The model under review builds one solid part; all positions refer to its coordinate system, in mm. Face numbers are marked on the shaded views. A direction names the side the tool comes from. Round coordinates to 2 decimals unless told otherwise and drop trailing zeros. Order: outer loops, then holes, each group sorted by start corner. A loop starts at its lowest first (then second) coordinate and runs counter-clockwise, first axis right, second up. Notation, with made-up numbers: M 21,6.5 L 32,6.5 A19 ccw 32,19.5 Z; hole C -21,36.25 d11. An arc over 180 degrees is marked long. Answer as a JSON object with one key per item and string values. Group by question number.
1) Consider section B-B, the plane z = 27.5. Write out the cut boundary in (x, y).
2) Consider section A-A, the plane y = -325.5. Write out the cut boundary in (x, z), then the cut area to 3 significant figures.
3) For the marked faces 1 and 2, list the 3-axis set-ups (+Z, -Z, +X, -X, +Y, -Y) from which the entire face can be reached by the end or side of a thin tool; tool diameter is ignored.
4) Insertion check: pin 1 Ø1 at (y, z) = (247.5, 47) entering from +X; pin 2 Ø4 at (x, y) = (27, 71.5) entering from -Z; pin 3 Ø8 at (x, y) = (7.5, -109.5) entering from -Z. Each pin has a flat end and moves straight along its axis. Give the tip position at first contact, or say it passes through.
5) Consider section C-C, the plane x = 48. Write out the cut boundary in (y, z).
6) To check wall thickness, follow line 1 (X direction, y = -69, z = 53); line 2 (Z direction, x = 9, y = -290); line 3 (X direction, y = -324.5, z = 4). State the ranges of each line that lie inside material, in increasing order.
```python
from build123d import *

# Parameters (mm, degrees)
F1_DEPTH = 482.6
F3_DEPTH = 6.351
F5_R     = 5.08
F4_R     = 7.14375
F6_DEPTH = 101.6


with BuildPart() as f1:
    # F0 (on Front) → F1 (new body, symmetric)
    with BuildSketch(Plane.XZ):
        Polygon((-6.35, 0), (0, 0), (0, 69.85), (69.85, 69.85), (69.85, 76.2), (-6.35, 76.2), align=None)
    extrude(amount=F1_DEPTH, both=True)

    # F2 (on Right) → F3 (cut, through all)
    with BuildSketch(Plane.YZ):
        Polygon((482.6, 0), (482.6, 69.85), (412.75, 0), align=None)
    extrude(amount=-F3_DEPTH, mode=Mode.SUBTRACT)

    # F5
    f5_edges = [f1.edges().sort_by_distance(p)[0] for p in [
        (0, 0, 69.85),
        (69.85, 0, 69.85),
        (0, -34.925, 0),
    ]]
    fillet(f5_edges, radius=F5_R)

    # F4 (on Top) → F6 (cut)
    with BuildSketch(Plane.XY):
        with Locations((31.806327, 104.775)):
            Circle(F4_R)
    extrude(amount=F6_DEPTH, mode=Mode.SUBTRACT)


solid = f1.part
```
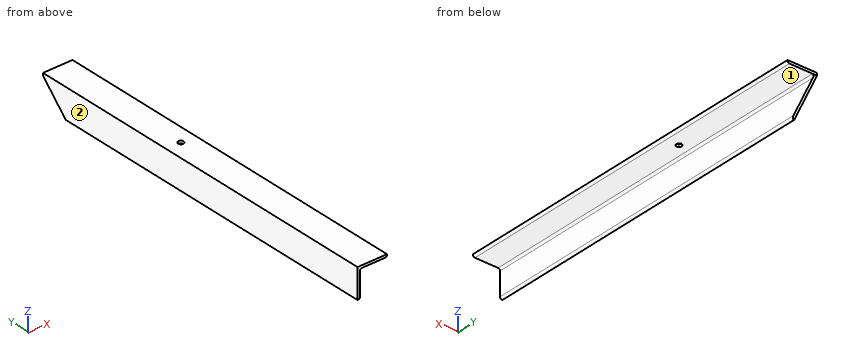
Results list:
{
 "1": {"outline": "M -6.35,-482.6 L 0,-482.6 L 0,440.25 L -6.35,440.25 Z"},
 "2": {"outline": "M -6.35,0 L -5.08,0 A5.08 ccw 0,5.08 L 0,64.77 A5.08 cw 5.08,69.85 L 64.77,69.85 A5.08 ccw 69.85,74.93 L 69.85,76.2 L -6.35,76.2 Z", "area": "922 mm^2"},
 "3": {"face 1": "-Z, +X, +Y, -Y", "face 2": "+Z, -Z, -X, +Y, -Y"},
 "4": {"pin 1": "x = 0", "pin 2": "z = 69.85", "pin 3": "z = 69.6"},
 "5": {"outline": "M -482.6,69.85 L 482.6,69.85 L 482.6,76.2 L -482.6,76.2 Z"},
 "6": {"line 1": "-6.35 to 0", "line 2": "69.85 to 76.2", "line 3": "-6.35 to -0.12"}
}
